```python
from build123d import *


with BuildPart() as part:
    # Sketch1 → Revolve1 (revolve)
    with BuildSketch(Plane.XY, mode=Mode.PRIVATE) as revolve1_sk:
        with BuildLine():
            Line((-3.7, 6), (3.7, 6))
            ThreePointArc((3.7, 6), (3.912132034, 6.087867966), (4, 6.3))
            Line((4, 6.3), (4, 8.75))
            Line((4, 8.75), (1.534411288, 8.75))
            ThreePointArc((1.534411288, 8.75), (0.396176489, 8.063947496), (-0.919738006, 8.25))
            Line((-0.919738006, 8.25), (-4, 8.25))
            Line((-4, 8.25), (-4, 6.3))
            ThreePointArc((-4, 6.3), (-3.912132034, 6.087867966), (-3.7, 6))
        make_face()
    revolve(revolve1_sk.sketch.rotate(Axis((4, 0, 0), (-1, 0, 0)), 270), axis=Axis((4, 0, 0), (-1, 0, 0)))


solid = part.part
```
Source: CAD feature listing. Evaluate the final solid. Frame: model axes, mm. A direction names the side the tool comes from. Round coordinates to 2 decimals unless told otherwise and drop trailing zeros. Loops run counter-clockwise (first coordinate to the right, second up) from the corner with the lowest first, then second, coordinate; pieces in that order, holes last.
(1) Access query for faces 1 (the cylindrical face through (-2.481, -8.054, -1.788)), 2 (the flat face through (4, -4, -6)). Directions: +Z, -Z, +X, -X, +Y, -Y. A direction counts if a zero-diameter tool reaches every point of the face in a straight line with its end or side. Return the directions, or none.
From the geometry:
face 1: -X
face 2: +Z, -Z, +X, +Y, -Y
(2) Contact query for flat-ended pins moving along their axis: pin 1 Ø3 at (x, z) = (0.5, 4) entering from -Y; pin 2 Ø1.5 at (x, y) = (3, -2) entering from +Z; pin 3 Ø2 at (x, y) = (2, 6.5) entering from -Z. Output: stop coordinate, or through.
From the geometry:
pin 1: stops at y = -8.25
pin 2: stops at z = 8.66
pin 3: stops at z = -6.81
(3) Pull-direction query (Y, two-part tool) for faces 3 (the flat face through (-4, -3, -6)), 4 (the cylindrical face through (0.052, 1.802, 5.723)), 5 (the cylindrical face through (2.75, -5.324, -6.944)); classes: +Y half, -Y half, draft (parallel to the pull), parting line (faces both ways), or undercut.
From the geometry:
face 3: draft
face 4: undercut
face 5: parting line
(4) Material intervals for probe 1 along Y at (x, z) = (-1.5, 0); probe 2 along Z at (x, y) = (-2.25, -0.25); probe 3 along Z at (x, y) = (-3.5, 1), sorted ascending.
From the geometry:
probe 1: y = -8.25 to -6, 6 to 8.25
probe 2: z = -8.25 to -5.99, 5.99 to 8.25
probe 3: z = -8.19 to -5.92, 5.92 to 8.19
(5) Section query A-A (y = 0). Output: boundary loops of the cut face in (x, z).
From the geometry:
outline: (-4, -8.25) - (-0.92, -8.25) arc R1.98 cw to (1.53, -8.75) - (4, -8.75) - (4, -6.3) arc R0.3 ccw to (3.7, -6) - (-3.7, -6) arc R0.3 ccw to (-4, -6.3) - close; (-4, 6.3) arc R0.3 ccw to (-3.7, 6) - (3.7, 6) arc R0.3 ccw to (4, 6.3) - (4, 8.75) - (1.53, 8.75) arc R1.98 cw to (-0.92, 8.25) - (-4, 8.25) - close
(6) Section query D-D (x = -1.5). Output: boundary loops of the cut face in (y, z).
From the geometry:
outline: circle Ø16.5 at (0, 0); hole circle Ø12 at (0, 0)
(7) Section query C-C (x = 2). Output: boundary loops of the cut face in (y, z).
From the geometry:
outline: circle Ø17.5 at (0, 0); hole circle Ø12 at (0, 0)
